```python
from build123d import *

# Parameters (mm, degrees)
BOSS_EXTRUDE1_DEPTH = 30
SKETCH5_W           = 48
SKETCH5_H           = 29
CUT_EXTRUDE1_DEPTH  = 29
SKETCH4_R           = 2.15
CUT_EXTRUDE2_DEPTH  = 58.879184514
SKETCH6_R           = 3.5
CUT_EXTRUDE3_DEPTH  = 55.460995217


with BuildPart() as part:
    # Sketch2 → Boss-Extrude1 (new, symmetric)
    with BuildSketch(Plane(origin=(0, 0, 0), x_dir=(0, 0, -1), z_dir=(1, 0, 0))):
        Polygon((0, 0), (35, 0), (35, 8), (8, 35), (0, 35), align=None)
    extrude(amount=BOSS_EXTRUDE1_DEPTH, both=True)

    # Sketch5 → Cut-Extrude1 (cut)
    with BuildSketch(Plane(origin=(0, 0, -35), x_dir=(-1, 0, 0), z_dir=(0, 0, -1))):
        with Locations((0, 20.5)):
            Rectangle(SKETCH5_W, SKETCH5_H)
    extrude(amount=-CUT_EXTRUDE1_DEPTH, mode=Mode.SUBTRACT)

    # Sketch4 → Cut-Extrude2 (cut, through all)
    with BuildSketch(Plane.XY):
        with Locations((-17.75, 20)):
            Circle(SKETCH4_R)
        with Locations((17.75, 20)):
            Circle(SKETCH4_R)
    extrude(amount=-CUT_EXTRUDE2_DEPTH, mode=Mode.SUBTRACT)

    # Sketch6 → Cut-Extrude3 (cut, through all)
    with BuildSketch(Plane(origin=(0, 6, 0), x_dir=(1, 0, 0), z_dir=(0, 1, 0))):
        with Locations(Location((0, 11, 0), (0, 0, 270))):
            Circle(SKETCH6_R)
        with Locations(Location((0, 29, 0), (0, 0, 90))):
            Circle(SKETCH6_R)
    extrude(amount=-CUT_EXTRUDE3_DEPTH, mode=Mode.SUBTRACT)


solid = part.part
```
Check sheet for the modelled part. Datum: model origin and axes. Units: mm. A direction names the side the tool comes from. Coordinates: 2 decimals unless noted, no trailing zeros. Order: outer loops, then holes, each group sorted by start corner. A loop starts at its lowest first (then second) coordinate and runs counter-clockwise, first axis right, second up. Notation, with made-up numbers: M 63,55 L 75,55 A14 ccw 75,82 Z; hole C -39,-37 d9. An arc over 180 degrees is marked long. One line per question, with ' | ' between items. Start each with the question number.
Item 1: Gauge pin test, flat ends, axial feed: P1, Ø14.5, axis at x = 11.5, z = -16, coming from the +Y side; P2, Ø7, axis at x = -17.75, y = 20, coming from the -Z side; P3, Ø12, axis at x = 21.5, z = -23.5, coming from the +Y side. Record the tip position at first contact, or that the pin passes through.
Item 2: Mould release check, pull along Z, two halves, no side actions. Record for faces 3 (the cylindrical face through (0.154, 3.042, -14.497)), 4 (the flat face through (-27, 21, -22)), 5 (the flat face through (0, 18, 0)), 6 (the flat face through (0, 6, -21)): pulls with the +Z half, pulls with the -Z half, needs draft (parallel to the pull), parting line crosses it, or undercut.
Item 3: Material ranges on line 1 (X direction, y = 27.5, z = -15); line 2 (Y direction, x = 17.75, z = -4.6); line 3 (X direction, y = 3.5, z = -29), recorded low to high.
Item 4: Sectioned sample at D-D on x = 0. Record the cut outline in (y, z), and give its area (3 significant figures).
Item 5: Sectioned sample at B-B on x = 17.75. Record the cut outline in (y, z), and give its area (3 significant figures).
Item 6: Access from +Z, -Z, +X, -X, +Y, -Y to the whole of each face (thin tool, end or side, straight path). Record for faces 1 (the cylindrical face through (17.28, 17.9, -2.96)), 2 (the flat face through (24, 17, -17)).
Item 7: Sectioned sample at A-A on y = 20. Record the cut outline in (x, z).
Item 8: Sectioned sample at C-C on z = -29. Record the cut outline in (x, y).
Answer below:
1) P1: stops at y = 6 | P2: stops at z = -6 | P3: stops at y = 24.95
2) face 3: undercut | face 4: pulls with the -Z half | face 5: pulls with the +Z half | face 6: needs draft
3) line 1: x = -30 to -24, 24 to 30 | line 2: y = 0 to 17.85, 22.15 to 35 | line 3: x = -30 to -3.5, 3.5 to 30
4) outline: M 0,-35 L 6,-35 L 6,-32.5 L 0,-32.5 Z; M 0,-25.5 L 6,-25.5 L 6,-14.5 L 0,-14.5 Z; M 0,-7.5 L 6,-7.5 L 6,-6 L 35,-6 L 35,0 L 0,0 Z | area: 300 mm^2
5) outline: M 0,-35 L 6,-35 L 6,-6 L 17.85,-6 L 17.85,0 L 0,0 Z; M 22.15,-6 L 35,-6 L 35,0 L 22.15,0 Z | area: 358 mm^2
6) face 1: +Z, -Z | face 2: -Z, +Y
7) outline: M -30,-23 L -24,-23 L -24,-6 L -19.9,-6 L -19.9,0 L -30,0 Z; M -15.6,-6 L 15.6,-6 L 15.6,0 L -15.6,0 Z; M 19.9,-6 L 24,-6 L 24,-23 L 30,-23 L 30,0 L 19.9,0 Z
8) outline: M -30,0 L -3.5,0 L -3.5,6 L -24,6 L -24,14 L -30,14 Z; M 3.5,0 L 30,0 L 30,14 L 24,14 L 24,6 L 3.5,6 Z
